Here's how the part is built. I have some questions about the finished solid (model axes, mm). A direction names the side the tool comes from. Give positions to 0.01 mm unless a question says otherwise; leave off trailing zeros. Loops run counter-clockwise (first coordinate to the right, second up) from the corner with the lowest first, then second, coordinate; pieces in that order, holes last. Notation, with made-up numbers: (78, 29.5) - (121, 29.5) arc R15 ccw to (121, 36.5) - close; hole circle Ø6 at (23.25, -26.5). An arc over 180 degrees is marked (long way). Use a Markdown table: item, result.
from build123d import *

# Parameters (mm, degrees)
F0_R     = 1.5
F1_DEPTH = 35
F0_R_2   = 3
F2_DEPTH = 1.7
F4_DEPTH = 1.5
F5_SIZE  = 1.49999


# Not quite as in the source:
# - a fillet or chamfer is up to 0.001 mm smaller than in the source, because OpenCascade refuses the exact size


with BuildPart() as f1:
    # F0 (on Top) → F1 (new body)
    with BuildSketch(Plane.XY):
        Circle(F0_R)
    extrude(amount=-F1_DEPTH)

    # F0 (on Top) → F2 (join)
    with BuildSketch(Plane.XY):
        Circle(F0_R_2)
        Circle(F0_R, mode=Mode.SUBTRACT)
        Circle(F0_R)
    extrude(amount=F2_DEPTH)

    # F3 (on face) → F4 (cut)
    with BuildSketch(Plane.XY.offset(1.7)):
        Polygon((-0.5773502692, -1), (0.5773502692, -1), (1.1547005384, 0), (0.5773502692, 1), (-0.5773502692, 1), (-1.1547005384, 0), align=None)
    extrude(amount=-F4_DEPTH, mode=Mode.SUBTRACT)

    # F5 (size 1.5 in the source; OpenCascade refuses exactly that, so slightly less here)
    f5_edges = [f1.edges().sort_by_distance(p)[0] for p in [
        (-3, 0, 0),
    ]]
    chamfer(f5_edges, length=F5_SIZE)


solid = f1.part
(1) Suppose I cut it at B-B on z = -3. Write out the boundary of the cut face in (x, y).
A:
| item | result |
|---|---|
| outline | circle Ø3 at (0, 0) |
(2) Will these pins go through, and if not, where does the flat tip stop? pin 1 (1 mm diameter, centred on x = -2, y = -2, fed in from -Z); pin 2 (1 mm diameter, centred on y = -1, z = -14.5, fed in from -X).
A:
| item | result |
|---|---|
| pin 1 | z = 0.83 |
| pin 2 | x = -1.41 |
(3) On a 3-axis mill with a long thin cutter (end or side, diameter ignored), from which of +Z, -Z, +X, -X, +Y, -Y can I reach the whole of each face in a straight line? I mean faces 1 (the face through (0, 1, 1)), 2 (the face through (0, -1.3, 1.7)). Say none if no direction works.
A:
| item | result |
|---|---|
| face 1 | +Z |
| face 2 | +Z, +X, -X, +Y, -Y |
(4) If I drill on line 1 (Z direction, x = -0.05, y = -0.5); line 2 (Y direction, x = 0.1, z = -9.5); line 3 (X direction, y = 0.35, z = -14.5), over which ranges is the centre line in solid material (lowest first)?
A:
| item | result |
|---|---|
| line 1 | -35 to 0.2 |
| line 2 | -1.5 to 1.5 |
| line 3 | -1.46 to 1.46 |
(5) We'd pull the mould along Y, two halves only. Please class faces 3 (the face through (0, 0, -35)), 4 (the face through (-1.5, 0.07, -17.26)), 5 (the face through (-0.87, -0.49, 0.96)): pulls with the +Y half, pulls with the -Y half, needs draft (parallel to the pull), parting line crosses it, or undercut.
A:
| item | result |
|---|---|
| face 3 | needs draft |
| face 4 | parting line crosses it |
| face 5 | undercut |
